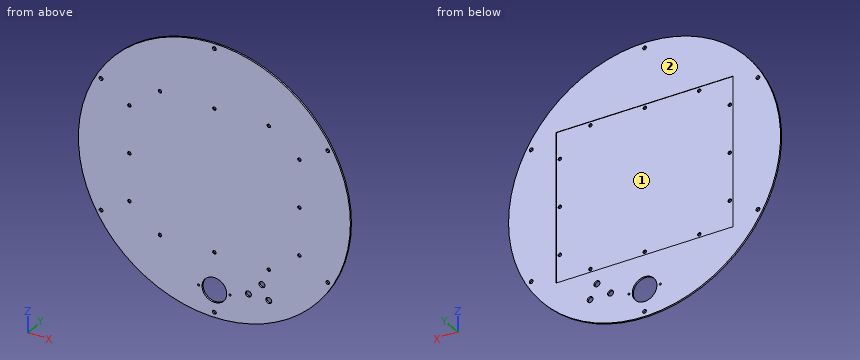
```python
from build123d import *

# Parameters (mm, degrees)
SKETCH1_R                = 508
COVER_DEPTH              = 6.35
COVER_B_C_D              = 14.2875
SKETCH3_W                = 660.4
SKETCH3_H                = 558.8
COVER_HATCH_DEPTH        = 1.5875
COVER_HATCH_BOLT_HOLES_D = 12.7
SKETCH33_R               = 46.0375
COVER_HOLE_ONE_DEPTH     = 7.35
COVER_HOLE_ONE_B_C_D     = 7.9375
SKETCH65_R               = 11.1125
COVER_HOLE_SIX_DEPTH     = 7.35
SKETCH66_R               = 11.1125
COVER_HOLE_SEVEN_DEPTH   = 7.35
SKETCH67_R               = 11.1125
COVER_HOLE_EIGHT_DEPTH   = 7.35


with BuildPart() as part:
    # Sketch1 → Cover (new body)
    with BuildSketch(Plane(origin=(0, 0, 0), x_dir=(1, 0, 0), z_dir=(0, 1, 0))):
        Circle(SKETCH1_R)
    extrude(amount=-COVER_DEPTH)

    # Cover B.C. (through all)
    with Locations(Plane(origin=(0, 0, 0), x_dir=(-1, 0, 0), z_dir=(0, 1, 0))):
        with Locations((0, -488.95), (-423.44312118, -244.475), (-423.44312118, 244.475), (0, 488.95), (423.44312118, 244.475), (423.44312118, -244.475)):
            Hole(COVER_B_C_D / 2)

    # Sketch3 → Cover Hatch (cut)
    with BuildSketch(Plane(origin=(0, 0, 0), x_dir=(-1, 0, 0), z_dir=(0, 1, 0))):
        Rectangle(SKETCH3_W, SKETCH3_H)
    extrude(amount=-COVER_HATCH_DEPTH, mode=Mode.SUBTRACT)

    # Cover Hatch Bolt Holes (through all)
    with Locations(Plane(origin=(0, -1.5875, 0), x_dir=(1, 0, 0), z_dir=(0, 1, 0))):
        with Locations((-317.5, 177.8), (-317.5, 0), (-317.5, -177.8), (317.5, -177.8), (317.5, 0), (317.5, 177.8), (-203.2, 266.7), (0, 266.7), (203.2, 266.7), (203.2, -266.7), (0, -266.7), (-203.2, -266.7)):
            Hole(COVER_HATCH_BOLT_HOLES_D / 2)

    # Sketch33 → Cover Hole One (cut, through all)
    with BuildSketch(Plane(origin=(0, 0, 0), x_dir=(1, 0, 0), z_dir=(0, 1, 0))):
        with Locations((0, 406.4)):
            Circle(SKETCH33_R)
    extrude(amount=-COVER_HOLE_ONE_DEPTH, mode=Mode.SUBTRACT)

    # Cover Hole One B.C. (through all)
    with Locations(Plane(origin=(0, 0, 0), x_dir=(1, 0, 0), z_dir=(0, 1, 0))):
        with Locations((-58.7375, 406.4), (58.7375, 406.4)):
            Hole(COVER_HOLE_ONE_B_C_D / 2)

    # Sketch65 → Cover Hole Six (cut, through all)
    with BuildSketch(Plane(origin=(0, 0, 0), x_dir=(1, 0, 0), z_dir=(0, 1, 0))):
        with Locations((127, 381)):
            Circle(SKETCH65_R)
    extrude(amount=-COVER_HOLE_SIX_DEPTH, mode=Mode.SUBTRACT)

    # Sketch66 → Cover Hole Seven (cut, through all)
    with BuildSketch(Plane(origin=(0, 0, 0), x_dir=(1, 0, 0), z_dir=(0, 1, 0))):
        with Locations((203.2, 381)):
            Circle(SKETCH66_R)
    extrude(amount=-COVER_HOLE_SEVEN_DEPTH, mode=Mode.SUBTRACT)

    # Sketch67 → Cover Hole Eight (cut, through all)
    with BuildSketch(Plane(origin=(0, 0, 0), x_dir=(1, 0, 0), z_dir=(0, 1, 0))):
        with Locations((177.8, 330.2)):
            Circle(SKETCH67_R)
    extrude(amount=-COVER_HOLE_EIGHT_DEPTH, mode=Mode.SUBTRACT)


solid = part.part
```
Source: CAD feature listing. Evaluate the final solid. Frame: model axes, mm. Face numbers are marked on the shaded views. Give positions to 0.01 mm unless a question says otherwise; leave off trailing zeros. Order: outer loops, then holes, each group sorted by start corner. A loop starts at its lowest first (then second) coordinate and runs counter-clockwise, first axis right, second up.
(1) Section query A-A (y = -4.75). State how many separate pieces and enclosed holes the cut face has, plus the area to 3 significant figures.
(2) Section query D-D (z = 425). Return the cut outline in (x, y), plus the area to 3 significant figures.
(3) Pull-direction query (X, two-part tool) for the marked faces 1 and 2; classes: +X half, -X half, draft (parallel to the pull), parting line (faces both ways), or undercut.
(4) Material intervals for line 1 along X through (y, z) = (-2.75, -266.7); line 2 along Z through (x, y) = (124, -1.25); line 3 along X through (y, z) = (-3.5, -267), sorted ascending.
(5) Section query B-B (z = -135.5). Return the cut outline in (x, y), plus the area to 3 significant figures.
(6) Contact query for flat-ended pins moving along their axis: P1, Ø3, axis at y = -5.5, z = -259.5, coming from the +X side; P2, Ø20.5, axis at x = -317.5, z = 0, coming from the +Y side; P3, Ø2, axis at y = -1, z = -122, coming from the -X side; P4, Ø10, axis at x = 0, z = 266.7, coming from the -Y side. Output: stop coordinate, or through.
(7) Section query C-C (x = -98). Return the cut outline in (y, z), plus the area to 3 significant figures.
Outcome:
1. separate pieces: 1
1. enclosed holes: 24
1. area: 800,000 mm2
2. outline: (-278.28, -6.35) - (278.28, -6.35) - (278.28, 0) - (-278.28, 0) - close
2. area: 3,530 mm2
3. face 1: undercut
3. face 2: draft
4. line 1: x = -432.36 to -209.55, -196.85 to -6.35, 6.35 to 196.85, 209.55 to 432.36
4. line 2: z = -492.63 to -391.7, -370.3 to -279.4, 279.4 to 492.63
4. line 3: x = -432.17 to -209.54, -196.86 to -6.34, 6.34 to 196.86, 209.54 to 432.17
5. outline: (-489.6, -6.35) - (489.6, -6.35) - (489.6, 0) - (330.2, 0) - (330.2, -1.59) - (-330.2, -1.59) - (-330.2, 0) - (-489.6, 0) - close
5. area: 5,170 mm2
6. P1: stops at x = 437.61
6. P2: stops at y = -1.59
6. P3: stops at x = -493.38
6. P4: passes through
7. outline: (-6.35, -498.46) - (0, -498.46) - (0, -279.4) - (-1.59, -279.4) - (-1.59, 279.4) - (0, 279.4) - (0, 498.46) - (-6.35, 498.46) - close
7. area: 5,440 mm2
